```python
from build123d import *

# Parameters (mm, degrees)
ESQUISSE3_W             = 63.5
ESQUISSE3_H             = 23.468408113
ESQUISSE3_R             = 1
BOSS_EXTRU_1_DEPTH      = 4
CONG_1_R                = 3
ESQUISSE3_3_R           = 1
ESQUISSE3_3_W           = 33.02
ESQUISSE3_3_H           = 4
ESQUISSE3_3_W_2         = 114.3
ENL_V_MAT_EXTRU_1_DEPTH = 1.5


with BuildPart() as part:
    # Esquisse3 → Boss.-Extru.1 (new body)
    with BuildSketch(Plane(origin=(0, 0, 0), x_dir=(1, 0, 0), z_dir=(0, 1, 0))):
        Polygon((-57.15, -30.5), (-16.51, -30.5), (-16.51, -61.4), (16.51, -61.4), (16.51, -30.5), (57.15, -30.5), (57.15, 30.5), (-57.15, 30.5), align=None)
        with Locations((0, -14.765795944)):
            Rectangle(ESQUISSE3_W, ESQUISSE3_H, mode=Mode.SUBTRACT)
        with Locations(Location((0, -28.5, 0), (0, 0, 270))):
            Circle(ESQUISSE3_R, mode=Mode.SUBTRACT)
        with Locations(Location((50, -28.5, 0), (0, 0, 270))):
            Circle(ESQUISSE3_R, mode=Mode.SUBTRACT)
        with Locations(Location((-50, -28.5, 0), (0, 0, 270))):
            Circle(ESQUISSE3_R, mode=Mode.SUBTRACT)
        with Locations(Location((50, 28.5, 0), (0, 0, 270))):
            Circle(ESQUISSE3_R, mode=Mode.SUBTRACT)
        with Locations(Location((-50, 28.5, 0), (0, 0, 270))):
            Circle(ESQUISSE3_R, mode=Mode.SUBTRACT)
        with Locations(Location((0, 28.5, 0), (0, 0, 270))):
            Circle(ESQUISSE3_R, mode=Mode.SUBTRACT)
        with Locations(Location((10, -59.4, 0), (0, 0, 270))):
            Circle(ESQUISSE3_R, mode=Mode.SUBTRACT)
        with Locations(Location((-10, -59.4, 0), (0, 0, 270))):
            Circle(ESQUISSE3_R, mode=Mode.SUBTRACT)
    extrude(amount=BOSS_EXTRU_1_DEPTH)

    # Cong_1
    cong_1_edges = [part.edges().sort_by_distance(p)[0] for p in [
        (-57.15, 2, 30.5),
        (-57.15, 2, -30.5),
        (57.15, 2, -30.5),
        (57.15, 2, 30.5),
        (16.51, 2, 30.5),
        (16.51, 2, 61.4),
        (-16.51, 2, 61.4),
        (-16.51, 2, 30.5),
        (31.75, 2, 26.5),
        (31.75, 2, 3.031591887),
        (-31.75, 2, 3.031591887),
        (-31.75, 2, 26.5),
    ]]
    fillet(cong_1_edges, radius=CONG_1_R)

    # Esquisse3_3 → Enl_v. mat.-Extru.1 (cut)
    # profile 1 of 3: a face of its own
    with BuildSketch(Plane(origin=(0, 0, 0), x_dir=(1, 0, 0), z_dir=(0, 1, 0))):
        Polygon((-31.75, -26.5), (-57.15, -26.5), (-57.15, -30.5), (-16.51, -30.5), (16.51, -30.5), (57.15, -30.5), (57.15, -26.5), (31.75, -26.5), align=None)
        with Locations(Location((-50, -28.5, 0), (0, 0, 270))):
            Circle(ESQUISSE3_3_R, mode=Mode.SUBTRACT)
        with Locations(Location((0, -28.5, 0), (0, 0, 270))):
            Circle(ESQUISSE3_3_R, mode=Mode.SUBTRACT)
        with Locations(Location((50, -28.5, 0), (0, 0, 270))):
            Circle(ESQUISSE3_3_R, mode=Mode.SUBTRACT)
    # profile 2 of 3: a face of its own
    with BuildSketch(Plane(origin=(0, 0, 0), x_dir=(1, 0, 0), z_dir=(0, 1, 0))):
        with Locations((0, -59.4)):
            Rectangle(ESQUISSE3_3_W, ESQUISSE3_3_H)
        with Locations(Location((-10, -59.4, 0), (0, 0, 270))):
            Circle(ESQUISSE3_3_R, mode=Mode.SUBTRACT)
        with Locations(Location((10, -59.4, 0), (0, 0, 270))):
            Circle(ESQUISSE3_3_R, mode=Mode.SUBTRACT)
    # profile 3 of 3: a face of its own
    with BuildSketch(Plane(origin=(0, 0, 0), x_dir=(1, 0, 0), z_dir=(0, 1, 0))):
        with Locations((0, 28.5)):
            Rectangle(ESQUISSE3_3_W_2, ESQUISSE3_3_H)
        with Locations(Location((-50, 28.5, 0), (0, 0, 270))):
            Circle(ESQUISSE3_3_R, mode=Mode.SUBTRACT)
        with Locations(Location((0, 28.5, 0), (0, 0, 270))):
            Circle(ESQUISSE3_3_R, mode=Mode.SUBTRACT)
        with Locations(Location((50, 28.5, 0), (0, 0, 270))):
            Circle(ESQUISSE3_3_R, mode=Mode.SUBTRACT)
    extrude(amount=ENL_V_MAT_EXTRU_1_DEPTH, mode=Mode.SUBTRACT)


solid = part.part
```
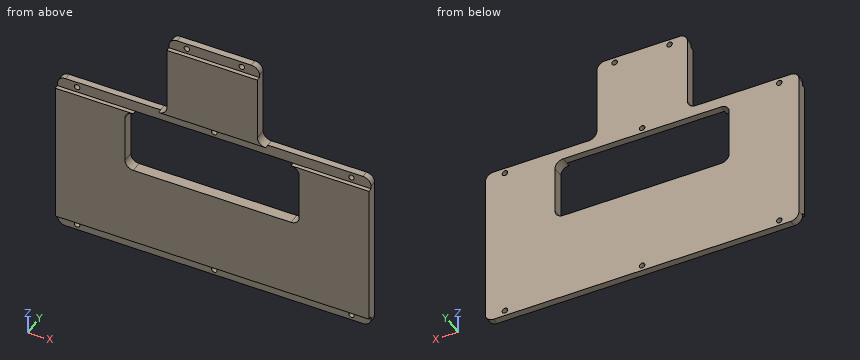
Work out the finished part from the listing and answer in its coordinate system (mm). Give positions to 0.01 mm unless a question says otherwise; leave off trailing zeros. Loops run counter-clockwise (first coordinate to the right, second up) from the corner with the lowest first, then second, coordinate; pieces in that order, holes last. Notation, with made-up numbers: (69.5, 43) - (126.5, 43) arc R18 cw to (126.5, 60) - close; hole circle Ø5 at (74.25, 28). An arc over 180 degrees is marked (long way). Use CSV: the item, a comma, the result in double quotes. Start each with the question number.
(1) Each of these flat-tipped pins is pushed along its axis until it touches: pin 1 (3 mm diameter, centred on x = 1.5, z = 59.5, fed in from -Y); pin 2 (2 mm diameter, centred on y = 3.5, z = 49, fed in from -X); pin 3 (0.8 mm diameter, centred on x = 49.5, y = 0.5, fed in from +Z); pin 4 (1.6 mm diameter, centred on x = 50, z = -28.5, fed in from -Y). Where does it stop, or does it pass through?
(2) Find section C-C, the plane y = 2.9. Count the separate pieces of the cut face and the enclosed holes in it, plus the area to 3 significant figures.
(3) Find section B-B, the plane z = 17. Determine the outline of the cut face in (x, y), plus the area to 3 significant figures.
(4) Find the intervals of material crossed by L1, parallel to Z at x = 8.5, y = 0.4; L2, parallel to Z at x = -29, y = 3.45; L3, parallel to X at y = 1.45, z = 9, in increasing order.
(5) Find section A-A, the plane x = -6.5. Determine the outline of the cut face in (y, z), plus the area to 3 significant figures.
(6) Find section D-D, the plane x = -40.5. Determine the outline of the cut face in (y, z), plus the area to 3 significant figures.
Results found:
1,pin 1,"y = 1.5"
1,pin 2,"x = -16.51"
1,pin 3,"z = 26.5"
1,pin 4,"through"
2,separate pieces,"1"
2,enclosed holes,"9"
2,area,"6,480 mm^2"
3,outline,"(-57.15, 0) - (-31.75, 0) - (-31.75, 4) - (-57.15, 4) - close; (31.75, 0) - (57.15, 0) - (57.15, 4) - (31.75, 4) - close"
3,area,"203 mm^2"
4,L1,"-26.5 to 3.03, 30.5 to 57.4"
4,L2,"-30.5 to 3.04, 26.49 to 30.5"
4,L3,"-57.15 to -31.75, 31.75 to 57.15"
5,outline,"(0, -26.5) - (1.5, -26.5) - (1.5, -30.5) - (4, -30.5) - (4, 3.03) - (0, 3.03) - close; (0, 30.5) - (1.5, 30.5) - (1.5, 26.5) - (4, 26.5) - (4, 61.4) - (1.5, 61.4) - (1.5, 57.4) - (0, 57.4) - close"
5,area,"256 mm^2"
6,outline,"(0, -26.5) - (1.5, -26.5) - (1.5, -30.5) - (4, -30.5) - (4, 30.5) - (1.5, 30.5) - (1.5, 26.5) - (0, 26.5) - close"
6,area,"232 mm^2"
